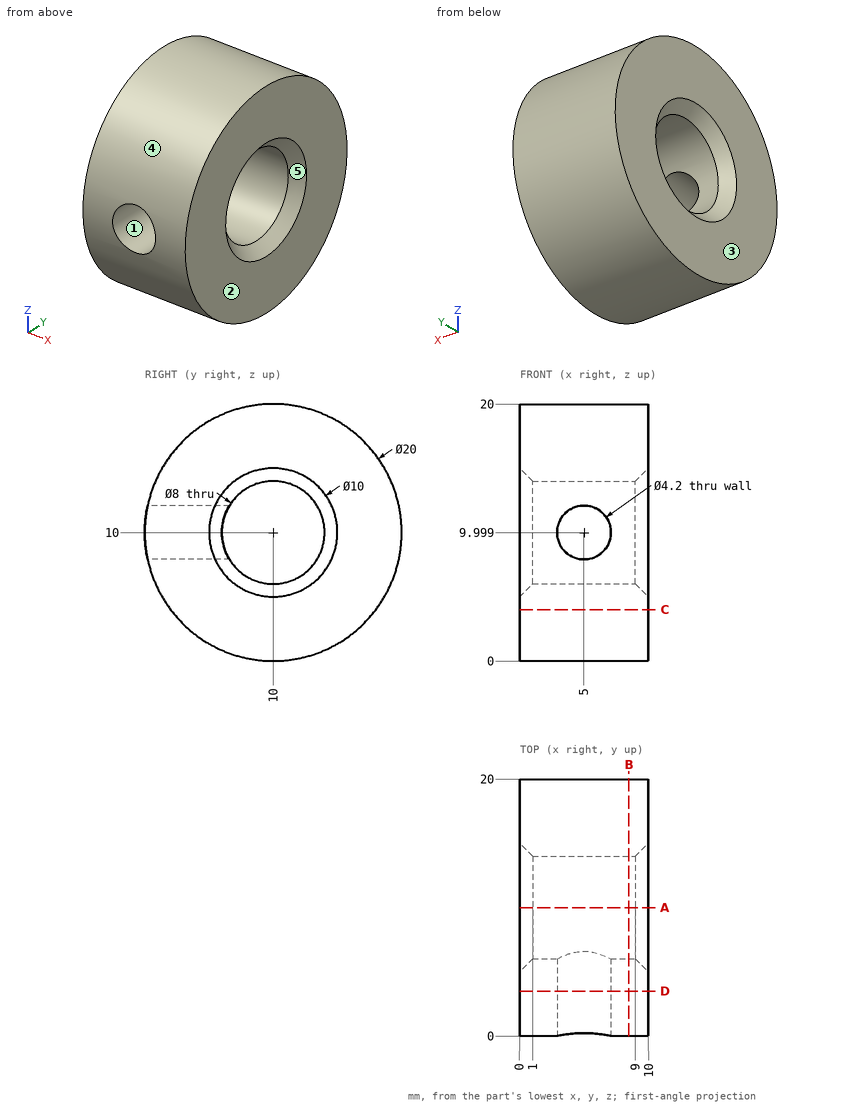
For this review, use the dimensioned drawing (mm, ordinates from the lowest corner) and the shaded views. A direction names the side the tool comes from. Round coordinates to 2 decimals unless told otherwise and drop trailing zeros. Order: outer loops, then holes, each group sorted by start corner. A loop starts at its lowest first (then second) coordinate and runs counter-clockwise, first axis right, second up.
1) Consider section B-B (x = 8.5). State the section outline as (y, z) points.
The answers:
outline: circle Ø20 at (10, 10); hole circle Ø8 at (10, 10)
2) For L1, parallel to Z at x = 4.5, y = 3.5; L2, parallel to Y at x = 6.75, z = 10; L3, parallel to Z at x = 5, y = 4.75, list the stretches that pass through material, from the lowest coordinate up.
The answers:
L1: z = 2.4 to 7.96, 12.04 to 17.6
L2: y = 14 to 20
L3: z = 1.49 to 7.9, 12.1 to 18.51
3) Clearance check with a flat-ended pin moving along its axis: pin 1 Ø10.5 at (y, z) = (10, 10) entering from +X. State where the tip first meets the part, or that it passes through.
The answers:
pin 1: stops at x = 10
4) Machinability: for the marked faces 1 and 2, which of the approach directions +Z, -Z, +X, -X, +Y, -Y give a long, thin tool a straight path to every point of the face, cutting with its end or side? Answer none if there is none.
The answers:
face 1: -Y
face 2: +Z, -Z, +X, +Y, -Y
5) Consider section D-D (y = 3.5). State the section outline as (x, z) points, plus the area to 3 significant figures.
The answers:
outline: (0, 2.4) - (10, 2.4) - (10, 17.6) - (0, 17.6) - close; hole circle Ø4.2 at (5, 10)
area: 138 mm2
6) Consider section C-C (z = 4). State the section outline as (x, y) points, plus the area to 3 significant figures.
The answers:
outline: (0, 2) - (10, 2) - (10, 18) - (0, 18) - close
area: 160 mm2
7) Draft analysis for pull direction Y (two halves, no side actions). For the marked faces 3, 4 and 5, state which applies: released by +Y, released by -Y, zero draft, split by the parting line, or undercut.
The answers:
face 3: zero draft
face 4: split by the parting line
face 5: undercut
8) Consider section A-A (y = 10). State the section outline as (x, z) points, plus the area to 3 significant figures.
The answers:
outline: (0, 0) - (10, 0) - (10, 5) - (9, 6) - (1, 6) - (0, 5) - close; (0, 15) - (1, 14) - (9, 14) - (10, 15) - (10, 20) - (0, 20) - close
area: 118 mm2
